from build123d import *

# Parameters (mm, degrees)
F1_DEPTH = 1.9
F0_W     = 1.5
F0_H     = 18.6
F2_DEPTH = 3
F3_DEPTH = 1.45
F4_DEPTH = 0.45


with BuildPart() as f1:
    # F0 (on Top) → F1 (new body)
    with BuildSketch(Plane.XY):
        with BuildLine():
            Line((-15.7, 0), (-5.8, 0))
            Line((-5.8, 0), (-5.8, 1))
            ThreePointArc((-5.8, 1), (-4.9, 1.9), (-4, 1))
            Line((-4, 1), (-3, -14.567916))
            Line((-3, -14.567916), (-1, -13.067916))
            ThreePointArc((-1, -13.067916), (-1.638952, -11.564856), (-0.672094, -10.248561))
            Line((-0.672094, -10.248561), (-0.908519, -6.567916))
            Line((-0.908519, -6.567916), (-1.036988, -4.567916))
            Line((-1.036988, -4.567916), (-1.394642, 1))
            ThreePointArc((-1.394642, 1), (-0.986161, 1.986161), (0, 2.394642))
            ThreePointArc((0, 2.394642), (0.986161, 1.986161), (1.394642, 1))
            Line((1.394642, 1), (1.036988, -4.567916))
            Line((1.036988, -4.567916), (0.908519, -6.567916))
            Line((0.908519, -6.567916), (0.672094, -10.248561))
            ThreePointArc((0.672094, -10.248561), (1.638952, -11.564856), (1, -13.067916))
            Line((1, -13.067916), (3, -14.567916))
            Line((3, -14.567916), (4, 1))
            ThreePointArc((4, 1), (4.9, 1.9), (5.8, 1))
            Line((5.8, 1), (5.8, 0))
            Line((5.8, 0), (15.7, 0))
            Line((15.7, 0), (15.7, 18.6))
            Line((15.7, 18.6), (8.603879, 18.6))
            ThreePointArc((8.603879, 18.6), (7.744643, 14.852036), (5.338554, 11.852662))
            ThreePointArc((5.338554, 11.852662), (0, 9.996121), (-5.338553, 11.852662))
            ThreePointArc((-5.338553, 11.852662), (-7.744643, 14.852036), (-8.603879, 18.6))
            Line((-8.603879, 18.6), (-15.7, 18.6))
            Line((-15.7, 18.6), (-15.7, 0))
        make_face()
        with BuildLine():
            ThreePointArc((-4.2, 9.5), (-9.900402, 8.19316), (-5.338553, 11.852662))
            ThreePointArc((-5.338553, 11.852662), (-4.499598, 10.80684), (-4.2, 9.5))
        make_face(mode=Mode.SUBTRACT)
        with BuildLine():
            ThreePointArc((10.2, 9.5), (5.89316, 6.799598), (5.338554, 11.852662))
            ThreePointArc((5.338554, 11.852662), (8.50684, 12.200402), (10.2, 9.5))
        make_face(mode=Mode.SUBTRACT)
        with BuildLine():
            Line((0, 18.6), (-8.603879, 18.6))
            ThreePointArc((-8.603879, 18.6), (-7.744643, 14.852036), (-5.338553, 11.852662))
            ThreePointArc((-5.338553, 11.852662), (0, 9.996121), (5.338554, 11.852662))
            ThreePointArc((5.338554, 11.852662), (7.744643, 14.852036), (8.603879, 18.6))
            Line((8.603879, 18.6), (0, 18.6))
        make_face()
        with BuildLine():
            ThreePointArc((8.603879, 18.6), (0, 27.203879), (-8.603879, 18.6))
            Line((-8.603879, 18.6), (0, 18.6))
            Line((0, 18.6), (8.603879, 18.6))
        make_face()
    extrude(amount=F1_DEPTH)

    # F0 (on Top) → F2 (join)
    with BuildSketch(Plane.XY):
        with Locations((-16.45, 9.3)):
            Rectangle(F0_W, F0_H)
        with Locations((16.45, 9.3)):
            Rectangle(F0_W, F0_H)
    extrude(amount=F2_DEPTH)

    # F0 (on Top) → F3 (join)
    with BuildSketch(Plane.XY):
        Polygon((-1.036988, -4.567916), (-0.908519, -6.567916), (0.908519, -6.567916), (1.036988, -4.567916), align=None)
    extrude(amount=F3_DEPTH)

    # F0 (on Top) → F4 (cut)
    with BuildSketch(Plane.XY):
        Polygon((-1.036988, -4.567916), (-0.908519, -6.567916), (0.908519, -6.567916), (1.036988, -4.567916), align=None)
    extrude(amount=F4_DEPTH, mode=Mode.SUBTRACT)


solid = f1.part
Check sheet for the modelled part. Datum: model origin and axes. Units: mm. A direction names the side the tool comes from. Coordinates: 2 decimals unless noted, no trailing zeros. Loops run counter-clockwise (first coordinate to the right, second up) from the corner with the lowest first, then second, coordinate; pieces in that order, holes last. Notation, with made-up numbers: (-31, 5) -> (10, 5) arc R16 cw to (10, 31) -> close; hole circle Ø8 at (-16, 21). An arc over 180 degrees is marked (long way). Answer in a Markdown table with one row per item.
1. Sectioned sample at B-B, the plane x = 4.9. Record the boundary of the cut face in (y, z), then the cut area to 3 significant figures.
Check values:
| item | result |
|---|---|
| outline | (1.9, 0) -> (7.57, 0) -> (7.57, 1.9) -> (1.9, 1.9) -> close; (11.43, 0) -> (25.67, 0) -> (25.67, 1.9) -> (11.43, 1.9) -> close |
| area | 37.8 mm2 |
2. Release check for a two-part mould opening along Y. For faces 1 (the face through (3.493, -6.893, 0.937)), 2 (the face through (5.8, 0.5, 0.9)), 3 (the face through (0, -6, 0.45)) record: released by +Y, released by -Y, zero draft, split by the parting line, or undercut.
Check values:
| item | result |
|---|---|
| face 1 | released by -Y |
| face 2 | zero draft |
| face 3 | undercut |
3. Access from +Z, -Z, +X, -X, +Y, -Y to the whole of each face (thin tool, end or side, straight path). Record for faces 4 (the face through (-15.7, 9.2, 2.4)), 5 (the face through (0, -6.568, 1)), 6 (the face through (-13, 18.6, 1)).
Check values:
| item | result |
|---|---|
| face 4 | +Z, +Y, -Y |
| face 5 | +Z, -Z |
| face 6 | +Z, -Z, -X, +Y |
4. Material ranges on line 1 along X through (y, z) = (9.5, 1.35); line 2 along X through (y, z) = (3.5, 2.05); line 3 along Z through (x, y) = (10.5, 18.5), recorded low to high. Write a range as [from, to].
Check values:
| item | result |
|---|---|
| line 1 | x = [-17.2, -10.2], [-4.2, 4.2], [10.2, 17.2] |
| line 2 | x = [-17.2, -15.7], [15.7, 17.2] |
| line 3 | z = [0, 1.9] |
5. Sectioned sample at D-D, the plane x = 11. Record the boundary of the cut face in (y, z), then the cut area to 3 significant figures.
Check values:
| item | result |
|---|---|
| outline | (0, 0) -> (18.6, 0) -> (18.6, 1.9) -> (0, 1.9) -> close |
| area | 35.3 mm2 |
6. Go/stop test with flat-tipped pins: pin 1 (2 mm diameter, centred on x = -7.5, y = 5, fed in from +Z); pin 2 (1.5 mm diameter, centred on x = -13, z = 1.5, fed in from -Y); pin 3 (1.1 mm diameter, centred on x = 0.5, z = 1, fed in from -Y). Record where each tip stops, or that it passes through.
Check values:
| item | result |
|---|---|
| pin 1 | stops at z = 1.9 |
| pin 2 | stops at y = 0 |
| pin 3 | stops at y = -13.11 |
7. Sectioned sample at A-A, the plane y = 5. Record the boundary of the cut face in (x, z).
Check values:
| item | result |
|---|---|
| outline | (-17.2, 0) -> (17.2, 0) -> (17.2, 3) -> (15.7, 3) -> (15.7, 1.9) -> (-15.7, 1.9) -> (-15.7, 3) -> (-17.2, 3) -> close |
8. Sectioned sample at C-C, the plane y = -7.5. Record the boundary of the cut face in (x, z).
Check values:
| item | result |
|---|---|
| outline | (-3.45, 0) -> (-0.85, 0) -> (-0.85, 1.9) -> (-3.45, 1.9) -> close; (0.85, 0) -> (3.45, 0) -> (3.45, 1.9) -> (0.85, 1.9) -> close |
